from build123d import *

# Parameters (mm, degrees)
SKETCH1_R             = 24.13
SKETCH1_R_2           = 20.955
BOSS_EXTRUDE1_DEPTH   = 15
SKETCH1_R_3           = 5.775
SKETCH1_R_4           = 2.6
BOSS_EXTRUDE1_2_DEPTH = 15
SKETCH3_W             = 3
SKETCH3_H             = 18.355
BOSS_EXTRUDE3_DEPTH   = 15
CIRPATTERN1_COUNT     = 6
SKETCH4_R             = 0.89
SKETCH5_W             = 5
SKETCH5_H             = 0.5
BOSS_EXTRUDE4_DEPTH   = 15


with BuildPart() as part:
    # Sketch1 → Boss-Extrude1 (new body)
    with BuildSketch(Plane.XY):
        Circle(SKETCH1_R)
        Circle(SKETCH1_R_2, mode=Mode.SUBTRACT)
    extrude(amount=BOSS_EXTRUDE1_DEPTH)



with BuildPart() as body_2:
    # Sketch1 → Boss-Extrude1 2 (new body)
    with BuildSketch(Plane.XY):
        Circle(SKETCH1_R_3)
        Circle(SKETCH1_R_4, mode=Mode.SUBTRACT)
    extrude(amount=BOSS_EXTRUDE1_2_DEPTH)


with BuildPart() as part_1:
    add(part.part)

    add(body_2.part)  # Boss-Extrude3 merges body 2
    # Sketch3 → Boss-Extrude3 (add)
    with BuildSketch(Plane(origin=(0, 0, 0), x_dir=(-1, 0, 0), z_dir=(0, 0, -1))):
        with Locations((0, 11.7775)):
            Rectangle(SKETCH3_W, SKETCH3_H)
    boss_extrude3 = extrude(amount=-BOSS_EXTRUDE3_DEPTH)

    # CirPattern1: Boss-Extrude3 ×6 about axis
    cirpattern1_axis = Axis((0, 0, 0), (0, 0, 1))
    for i in range(1, CIRPATTERN1_COUNT):
        add(boss_extrude3.rotate(cirpattern1_axis, i * 360 / CIRPATTERN1_COUNT))

    # Sketch4 → Cut-Revolve1 (revolve, cut)
    with BuildSketch(Plane(origin=(0, 0, 0), x_dir=(0, 0, -1), z_dir=(1, 0, 0)), mode=Mode.PRIVATE) as cut_revolve1_sk:
        with Locations((-12.5, 24.13)):
            Circle(SKETCH4_R)
        with Locations((-2.5, 24.13)):
            Circle(SKETCH4_R)
    revolve(cut_revolve1_sk.sketch.rotate(Axis((0, 0, 0), (0, 0, 1)), 90), axis=Axis((0, 0, 0), (0, 0, 1)), mode=Mode.SUBTRACT)

    # Sketch5 → Boss-Extrude4 (add)
    with BuildSketch(Plane.XY.offset(15)):
        with Locations((0, 2.35)):
            Rectangle(SKETCH5_W, SKETCH5_H)
    extrude(amount=-BOSS_EXTRUDE4_DEPTH)


solid = part_1.part
Verification items for the finished model (mm, model axes). A direction names the side the tool comes from. Give positions to 0.01 mm unless a question says otherwise; leave off trailing zeros. Write each loop counter-clockwise with the first axis right and the second up, starting at its lowest first coordinate (ties: lowest second). Pieces come first, ordered by that corner, then holes. Notation, with made-up numbers: M -9,-38 L 12,-38 A28 ccw 12,-19 Z; hole C 1.5,-34 d6. An arc over 180 degrees is marked long. Use CSV: the item, a comma, the result in double quotes.
1) Cross-section at C-C (z = 10.25). Enter the section's corners in (x, y) (3 decimals), plus the area to 3 significant figures.
Final values:
outline,"C 0,0 d48.26; hole M -18.851,-9.152 L -5.58,-1.489 A5.775 cw -5.58,1.489 L -18.851,9.152 A20.955 ccw Z; hole M -17.351,-11.75 A20.955 ccw -1.5,-20.901 L -1.5,-5.577 A5.775 cw -4.08,-4.087 Z; hole M -17.351,11.75 L -4.08,4.087 A5.775 cw -1.5,5.577 L -1.5,20.901 A20.955 ccw Z; hole M -1.533,2.1 A2.6 ccw long 1.533,2.1 Z; hole M 1.5,-20.901 A20.955 ccw 17.351,-11.75 L 4.08,-4.087 A5.775 cw 1.5,-5.577 Z; hole M 1.5,5.577 A5.775 cw 4.08,4.087 L 17.351,11.75 A20.955 ccw 1.5,20.901 Z; hole M 5.58,-1.489 L 18.851,-9.152 A20.955 ccw 18.851,9.152 L 5.58,1.489 A5.775 cw Z"
area,"808 mm²"
2) Access from +Z, -Z, +X, -X, +Y, -Y to the whole of each face (thin tool, end or side, straight path). Record for faces 4 (the face through (10.622, -7.865, 7.395)), 5 (the face through (5, -2, 15)).
Final values:
face 4,"+Z, -Z"
face 5,"+Z, +X, -X, +Y, -Y"
3) Cross-section at B-B (y = 0). Enter the section's corners in (x, z) (3 decimals).
Final values:
outline,"M -24.13,0 L -20.955,0 L -20.955,15 L -24.13,15 L -24.13,13.39 A0.89 cw -24.13,11.61 L -24.13,3.39 A0.89 cw -24.13,1.61 Z; M -5.775,0 L -2.6,0 L -2.6,15 L -5.775,15 Z; M 2.6,0 L 5.775,0 L 5.775,15 L 2.6,15 Z; M 20.955,0 L 24.13,0 L 24.13,1.61 A0.89 cw 24.13,3.39 L 24.13,11.61 A0.89 cw 24.13,13.39 L 24.13,15 L 20.955,15 Z"
4) Material ranges on line 1 along Y through (x, z) = (0, 10.75); line 2 along Y through (x, z) = (14, 6.75); line 3 along X through (y, z) = (2, 11.75), recorded low to high.
Final values:
line 1,"-24.13 to -2.6, 2.1 to 24.13"
line 2,"-19.65 to -15.59, -9.81 to -6.35, 6.35 to 9.81, 15.59 to 19.65"
line 3,"-23.57 to -20.86, -6.46 to -1.66, 1.66 to 6.46, 20.86 to 23.57"
5) Cross-section at A-A (x = 0). Enter the section's corners in (y, z), plus the area to 3 significant figures.
Final values:
outline,"M -24.13,0 L -2.6,0 L -2.6,15 L -24.13,15 L -24.13,13.39 A0.89 cw -24.13,11.61 L -24.13,3.39 A0.89 cw -24.13,1.61 Z; M 2.1,0 L 24.13,0 L 24.13,1.61 A0.89 cw 24.13,3.39 L 24.13,11.61 A0.89 cw 24.13,13.39 L 24.13,15 L 2.1,15 Z"
area,"648 mm²"
6) Cross-section at D-D (y = -19.5). State how many separate pieces and enclosed holes the cut face has, plus the area to 3 significant figures.
Final values:
separate pieces,"3"
enclosed holes,"0"
area,"232 mm²"
7) Go/stop test with flat-tipped pins: pin 1 Ø4.5 at (y, z) = (12.5, 10) entering from -X; pin 2 Ø2.5 at (x, z) = (-0.5, 4.5) entering from -Y; pin 3 Ø8 at (y, z) = (-11.5, 10) entering from -X. Record where each tip stops, or that it passes through.
Final values:
pin 1,"x = -21.84"
pin 2,"y = -24.13"
pin 3,"x = -22.93"
8) Release check for a two-part mould opening along Y. For faces 1 (the face through (12.97, 20.35, 14.18)), 2 (the face through (0, -5, 0)), 3 (the face through (1.5, 13, 7)) record: released by +Y, released by -Y, zero draft, split by the parting line, or undercut.
Final values:
face 1,"split by the parting line"
face 2,"zero draft"
face 3,"undercut"
